Verification items for the finished model (mm, model axes). Face numbers are marked on the shaded views. A direction names the side the tool comes from. Round coordinates to 2 decimals unless told otherwise and drop trailing zeros. Loops run counter-clockwise (first coordinate to the right, second up) from the corner with the lowest first, then second, coordinate; pieces in that order, holes last. Notation, with made-up numbers: (86.25, -10) -> (109.25, -10) arc R30 ccw to (109.25, 26) -> close; hole circle Ø3 at (-24, 35.5). An arc over 180 degrees is marked (long way). Use a Markdown table: item, result. Add a question column.
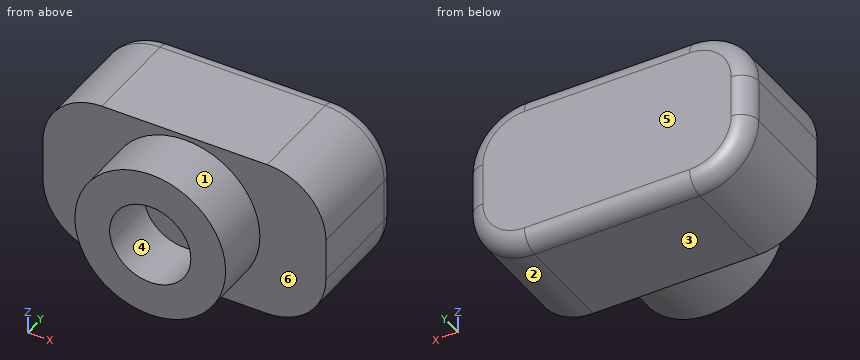
```python
from build123d import *

# Parameters (mm, degrees)
SKETCH1_R           = 3.25
BOSS_EXTRUDE1_DEPTH = 2.5
SKETCH2_R           = 1.75
CUT_EXTRUDE1_DEPTH  = 2.5
SKETCH3_W           = 12.2
SKETCH3_H           = 6.9
BOSS_EXTRUDE2_DEPTH = 5
FILLET1_R           = 2.54
FILLET2_R           = 0.75


with BuildPart() as part:
    # Sketch1 → Boss-Extrude1 (new body)
    with BuildSketch(Plane(origin=(0, 0, 0), x_dir=(1, 0, 0), z_dir=(0, 1, 0))):
        Circle(SKETCH1_R)
    extrude(amount=BOSS_EXTRUDE1_DEPTH)

    # Sketch2 → Cut-Extrude1 (cut)
    with BuildSketch(Plane.XZ):
        Circle(SKETCH2_R)
    extrude(amount=-CUT_EXTRUDE1_DEPTH, mode=Mode.SUBTRACT)

    # Sketch3 → Boss-Extrude2 (add)
    with BuildSketch(Plane(origin=(0, 2.5, 0), x_dir=(1, 0, 0), z_dir=(0, 1, 0))):
        Rectangle(SKETCH3_W, SKETCH3_H)
    extrude(amount=BOSS_EXTRUDE2_DEPTH)

    # Fillet1
    fillet1_edges = [part.edges().sort_by_distance(p)[0] for p in [
        (6.1, 5, 3.45),
        (6.1, 5, -3.45),
        (-6.1, 5, -3.45),
        (-6.1, 5, 3.45),
    ]]
    fillet(fillet1_edges, radius=FILLET1_R)

    # Fillet2
    fillet2_edges = [part.edges().sort_by_distance(p)[0] for p in [
        (-6.1, 7.5, 0),
        (0, 7.5, -3.45),
        (6.1, 7.5, 0),
        (0, 7.5, 3.45),
        (-5.356051224, 7.5, 2.706051224),
        (5.356051224, 7.5, 2.706051224),
        (5.356051224, 7.5, -2.706051224),
        (-5.356051224, 7.5, -2.706051224),
    ]]
    fillet(fillet2_edges, radius=FILLET2_R)


solid = part.part
```
1) Sectioned sample at A-A on y = 2.75. Enter the section's corners in (x, z), then the cut area to 3 significant figures.
2) Sectioned sample at C-C on z = 0. Enter the section's corners in (x, y), then the cut area to 3 significant figures.
3) Access from +Z, -Z, +X, -X, +Y, -Y to the whole of each face (thin tool, end or side, straight path). Record for the marked faces 5 and 6.
4) Go/stop test with flat-tipped pins: pin 1 (1.5 mm diameter, centred on x = -3, y = 1.5, fed in from -Z); pin 2 (1.8 mm diameter, centred on x = 0.5, z = 0, fed in from -Y). Record where each tip stops, or that it passes through.
5) Release check for a two-part mould opening along X. For the marked faces 1, 2, 3 and 4 record: released by +X, released by -X, zero draft, split by the parting line, or undercut.
6) Sectioned sample at D-D on x = 0. Enter the section's corners in (y, z).
7) Thickness scan on line 1 (Z direction, x = 0, y = 1.25); line 2 (Y direction, x = 5, z = 1); line 3 (X direction, y = 1.5, z = 1.25). Record the ranges inside material, lowest first.
8) Sectioned sample at B-B on x = 3. Enter the section's corners in (y, z), then the cut area to 3 significant figures.
Geometry results:
| question | item | result |
|---|---|---|
| 1 | outline | (-6.1, -0.91) arc R2.54 ccw to (-3.56, -3.45) -> (3.56, -3.45) arc R2.54 ccw to (6.1, -0.91) -> (6.1, 0.91) arc R2.54 ccw to (3.56, 3.45) -> (-3.56, 3.45) arc R2.54 ccw to (-6.1, 0.91) -> close |
| 1 | area | 78.6 mm^2 |
| 2 | outline | (-6.1, 2.5) -> (-3.25, 2.5) -> (-3.25, 0) -> (-1.75, 0) -> (-1.75, 2.5) -> (1.75, 2.5) -> (1.75, 0) -> (3.25, 0) -> (3.25, 2.5) -> (6.1, 2.5) -> (6.1, 6.75) arc R0.75 ccw to (5.35, 7.5) -> (-5.35, 7.5) arc R0.75 ccw to (-6.1, 6.75) -> close |
| 2 | area | 68.3 mm^2 |
| 3 | face 5 | +Z, -Z, +X, -X, +Y |
| 3 | face 6 | -Y |
| 4 | pin 1 | z = -2.35 |
| 4 | pin 2 | y = 2.5 |
| 5 | face 1 | split by the parting line |
| 5 | face 2 | released by +X |
| 5 | face 3 | zero draft |
| 5 | face 4 | undercut |
| 6 | outline | (0, -3.25) -> (2.5, -3.25) -> (2.5, -3.45) -> (6.75, -3.45) arc R0.75 ccw to (7.5, -2.7) -> (7.5, 2.7) arc R0.75 ccw to (6.75, 3.45) -> (2.5, 3.45) -> (2.5, 3.25) -> (0, 3.25) -> (0, 1.75) -> (2.5, 1.75) -> (2.5, -1.75) -> (0, -1.75) -> close |
| 7 | line 1 | -3.25 to -1.75, 1.75 to 3.25 |
| 7 | line 2 | 2.5 to 7.5 |
| 7 | line 3 | -3 to -1.22, 1.22 to 3 |
| 8 | outline | (0, -1.25) -> (2.5, -1.25) -> (2.5, -3.45) -> (6.75, -3.45) arc R0.75 ccw to (7.5, -2.7) -> (7.5, 2.7) arc R0.75 ccw to (6.75, 3.45) -> (2.5, 3.45) -> (2.5, 1.25) -> (0, 1.25) -> close |
| 8 | area | 40.5 mm^2 |
